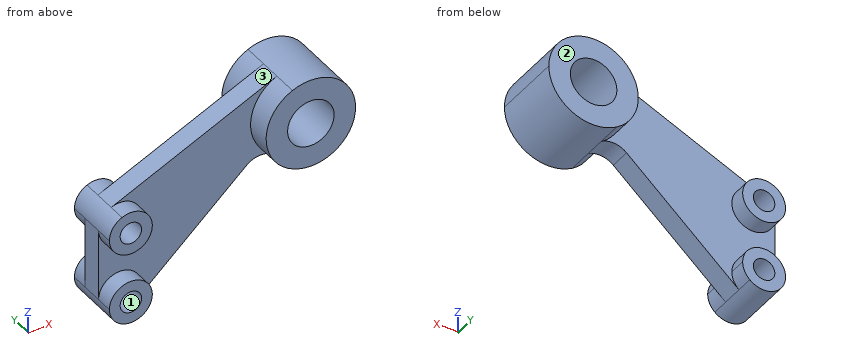
from build123d import *

# Parameters (mm, degrees)
F0_R     = 26.0096
F1_DEPTH = 40.005
F0_R_2   = 11.9888
F2_DEPTH = 31.496
F3_DEPTH = 11.9888


with BuildPart() as f1:
    # F0 (on Front) → F1 (new body, symmetric)
    with BuildSketch(Plane.XZ):
        with BuildLine():
            ThreePointArc((-25.898693, -42.784552), (24.55605, -43.569032), (50.0126, 0))
            ThreePointArc((50.0126, 0), (27.125002, 42.017787), (-20.589386, 45.577816))
            ThreePointArc((-20.589386, 45.577816), (-49.922564, 2.999628), (-25.898693, -42.784552))
        make_face()
        Circle(F0_R, mode=Mode.SUBTRACT)
    extrude(amount=F1_DEPTH, both=True)



with BuildPart() as f2:
    # F0 (on Front) → F2 (new body, symmetric)
    with BuildSketch(Plane.XZ):
        with BuildLine():
            ThreePointArc((-219.9894, -140.0048), (-205.782899, -161.917641), (-179.980017, -157.891659))
            ThreePointArc((-179.980017, -157.891659), (-174.073559, -149.801299), (-171.9834, -140.0048))
            ThreePointArc((-171.9834, -140.0048), (-195.9864, -116.0018), (-219.9894, -140.0048))
        make_face()
        with Locations((-195.9864, -140.0048)):
            Circle(F0_R_2, mode=Mode.SUBTRACT)
        with BuildLine():
            ThreePointArc((-171.9834, -59.9948), (-182.968052, -39.828823), (-205.868051, -38.120226))
            ThreePointArc((-205.868051, -38.120226), (-216.152377, -46.976452), (-219.9894, -59.9948))
            ThreePointArc((-219.9894, -59.9948), (-195.9864, -83.9978), (-171.9834, -59.9948))
        make_face()
        with Locations((-195.9864, -59.9948)):
            Circle(F0_R_2, mode=Mode.SUBTRACT)
    extrude(amount=F2_DEPTH, both=True)


with BuildPart() as f1_1:
    add(f1.part)

    add(f2.part)  # F3 merges F2
    # F0 (on Front) → F3 (join, symmetric)
    with BuildSketch(Plane.XZ):
        with BuildLine():
            ThreePointArc((-25.898693, -42.784552), (-49.922564, 2.999628), (-20.589386, 45.577816))
            Line((-20.589386, 45.577816), (-205.868051, -38.120226))
            ThreePointArc((-205.868051, -38.120226), (-182.968052, -39.828823), (-171.9834, -59.9948))
            ThreePointArc((-171.9834, -59.9948), (-195.9864, -83.9978), (-219.9894, -59.9948))
            Line((-219.9894, -59.9948), (-219.9894, -140.0048))
            ThreePointArc((-219.9894, -140.0048), (-195.9864, -116.0018), (-171.9834, -140.0048))
            ThreePointArc((-171.9834, -140.0048), (-174.073559, -149.801299), (-179.980017, -157.891659))
            Line((-179.980017, -157.891659), (-54.304779, -45.428869))
            ThreePointArc((-54.304779, -45.428869), (-40.537796, -39.422421), (-25.898693, -42.784552))
        make_face()
    extrude(amount=F3_DEPTH, both=True)


solid = f1_1.part
Input: part model. Units: mm. Frame: model coordinates. Face numbers are marked on the shaded views. Give positions to 0.01 mm unless a question says otherwise; leave off trailing zeros. Write each loop counter-clockwise with the first axis right and the second up, starting at its lowest first coordinate (ties: lowest second). Pieces come first, ordered by that corner, then holes. Notation, with made-up numbers: (59, -3) -> (93, -3) arc R26 ccw to (93, 20) -> close; hole circle Ø8 at (7, 61). An arc over 180 degrees is marked (long way). Use one line per item in the form item = value. Start each with the question number.
1) Section query D-D on x = -194.5. Return the cut outline in (y, z).
2) Section query A-A on x = 0. Return the cut outline in (y, z) (3 decimals), then the cut area to 3 significant figures.
3) Draft query along X for the marked faces 1, 2 and 3. Return one class per face: pulls with the +X half, pulls with the -X half, needs draft (parallel to the pull), parting line crosses it, or undercut.
4) Section query C-C on z = 14. Return the cut outline in (x, y) (3 decimals).
5) Pin query (flat end, axial travel): pin 1 (21.5 mm diameter, centred on x = -195.99, z = -59.99, fed in from -Y); pin 2 (12 mm diameter, centred on x = -155, z = -12.5, fed in from +Y); pin 3 (8 mm diameter, centred on y = 29.5, z = -81, fed in from -X); pin 4 (6 mm diameter, centred on x = -182, y = 25, fed in from -Z). Return the tip coordinate at first contact, or that it passes through.
6) Ray query, probe 1 along X at (y, z) = (30, 1.5); probe 2 along Z at (x, y) = (-188.5, -8); probe 3 along X at (y, z) = (31, -147.5). Return the intervals inside material, ascending. Write a range as from..to.
7) Section query B-B on y = -19.5. Return the cut outline in (x, z).
Outcome:
q1.outline = (-31.5, -163.96) -> (31.5, -163.96) -> (31.5, -151.9) -> (-31.5, -151.9) -> close; (-31.5, -128.11) -> (31.5, -128.11) -> (31.5, -116.05) -> (11.99, -116.05) -> (11.99, -83.95) -> (31.5, -83.95) -> (31.5, -71.89) -> (-31.5, -71.89) -> (-31.5, -83.95) -> (-11.99, -83.95) -> (-11.99, -116.05) -> (-31.5, -116.05) -> close; (-31.5, -48.1) -> (31.5, -48.1) -> (31.5, -36.04) -> (11.99, -36.04) -> (11.99, -32.98) -> (-11.99, -32.98) -> (-11.99, -36.04) -> (-31.5, -36.04) -> close
q2.outline = (-40.005, -50.013) -> (40.005, -50.013) -> (40.005, -26.01) -> (-40.005, -26.01) -> close; (-40.005, 26.01) -> (40.005, 26.01) -> (40.005, 50.013) -> (-40.005, 50.013) -> close
q2.area = 3,840 mm^2
q3.face_1 = undercut
q3.face_2 = needs draft
q3.face_3 = pulls with the -X half
q4.outline = (-90.492, -11.989) -> (-48.013, -11.989) -> (-48.013, -40.005) -> (-21.92, -40.005) -> (-21.92, 40.005) -> (-48.013, 40.005) -> (-48.013, 11.989) -> (-90.492, 11.989) -> close; (21.92, -40.005) -> (48.013, -40.005) -> (48.013, 40.005) -> (21.92, 40.005) -> close
q5.pin_1 = through
q5.pin_2 = 11.99
q5.pin_3 = -212.93
q5.pin_4 = -161.35
q6.probe_1 = -49.99..-25.97, 25.97..49.99
q6.probe_2 = -162.81..-149.37, -130.64..-69.36, -50.63..-30.27
q6.probe_3 = -218.79..-205.34, -186.63..-173.18
q7.outline = circle Ø48.01 at (-195.99, -59.99); (-179.98, -157.89) arc R24 ccw to (-171.98, -140) arc R24 ccw (long way) to start; circle Ø100.03 at (0, 0); hole circle Ø23.98 at (-195.99, -140); hole circle Ø23.98 at (-195.99, -59.99); hole circle Ø52.02 at (0, 0)
